Part model, mm, in its own coordinate system. Face numbers are marked on the shaded views. A direction names the side the tool comes from. Round coordinates to 2 decimals unless told otherwise and drop trailing zeros. Write each loop counter-clockwise with the first axis right and the second up, starting at its lowest first coordinate (ties: lowest second). Pieces come first, ordered by that corner, then holes.
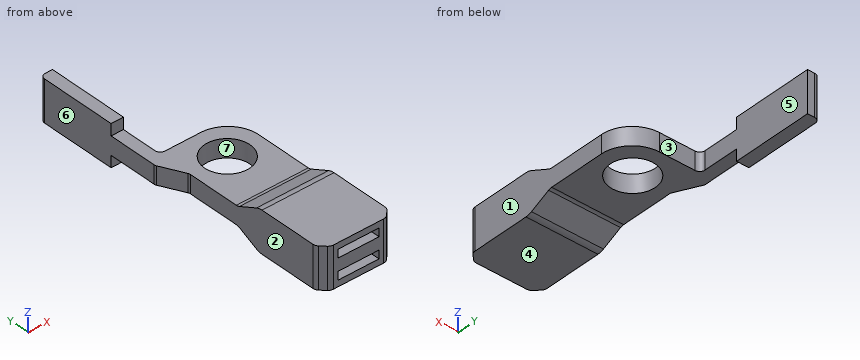
Autodesk Fusion 360 part; units mm, degrees
sketch "Sketch1" plane through (0, 0, 0) normal (0, 0, 1) x (1, 0, 0)
  circle A0 centre (0, 0) radius 11
  line L0 (-17.5, -72.5) -> (17.5, -72.5)
  line L1 (17.5, -72.5) -> (17.5, 17.5)
  line L2 (17.5, 17.5) -> (-17.5, 17.5)
  line L3 (-17.5, 17.5) -> (-17.5, -72.5)
  line L4 (-17.5, 76.6964) -> (-17.5, 51.5115)
  line L5 (-17.5, 51.5115) -> (-17.5, 17.5)
  line L6 (-23.5, 76.6964) -> (-23.5, 13.1317)
  line L7 (-23.5, 13.1317) -> (-17.5, 1.0512)
  line L8 (-17.5, 76.6964) -> (-23.5, 76.6964)
  dimension "d1" = 22
  dimension "d2" = 90
  dimension "d3" = 35
  dimension "d4" = 17.5
  dimension "d10" = 17.5
  dimension "d47" = 6
  dimension "d48" = 6
  dimension "d49" = 6
extrude "Extrude1" add sketch "Sketch1" along normal blind 20
sketch "Sketch4" plane through (-23.5, 0, 0) normal (-1, 0, 0) x (0, -1, 0)
  line L0 (-1.0512, 0) -> (72.5, 0)
  line L1 (72.5, 0) -> (72.5, 20)
  line L2 (72.5, 20) -> (-1.0512, 20)
  line L3 (72.5, 0) -> (72.5, 20)
  line L4 (37.5, 20) -> (25.7892, 14.3853)
  line L5 (25.7892, 14.3853) -> (-37.5, 14.3853)
  line L6 (-37.5, 14.3853) -> (-37.5, 5.6147)
  line L7 (-37.5, 5.6147) -> (25.7892, 5.6147)
  line L8 (25.7892, 5.6147) -> (37.5, 0)
  line L9 (72.5, 0) -> (72.5, 20)
  line L10 (-17.5, 0) -> (72.5, 0)
  line L11 (37.5, 20) -> (72.5, 20)
  line L12 (72.5, 0) -> (37.5, 0)
  line L13 (-37.5, 14.3853) -> (-37.5, 20)
  line L14 (-1.0512, 20) -> (-1.0512, 0)
  line L15 (-37.5, 0) -> (-37.5, 5.6147)
  line L16 (-1.0512, 20) -> (-1.0512, 0)
  line L17 (-76.6964, 0) -> (-13.1317, 0)
  line L18 (-13.1317, 0) -> (-13.1317, 20)
  line L19 (-13.1317, 20) -> (-76.6964, 20)
  line L20 (-76.6964, 20) -> (-76.6964, 0)
  line L21 (-13.1317, 20) -> (-1.0512, 20)
  dimension "d16" = 110
  dimension "d17" = 35
  dimension "d40" = 5.6147
  dimension "d41" = 8.7705
extrude "Extrude2" cut sketch "Sketch4" against normal blind 52 contours L0 L7 L8 L10 L14 L16 | L7 L10 L14 L16 L18 | L7 L10 L15 L17 L18 | L2 L4 L5 L14 L16 | L5 L14 L16 L18 L21 | L5 L13 L18 L19
chamfer "Chamfer1" distance 4 angle 45 2 edges at (-17.5, -72.5, 10) (17.5, -72.5, 10)
sketch "Sketch6" plane through (0, -72.5, 0) normal (0, -1, 0) x (1, 0, 0)
  line L0 (13.5, 0) -> (13.5, 20)
  line L1 (13.5, 20) -> (-13.5, 20)
  line L2 (-13.5, 20) -> (-13.5, 0)
  line L3 (-13.5, 0) -> (13.5, 0)
  line L4 (-10, 17) -> (10, 17)
  line L5 (10, 13) -> (-10, 13)
  line L6 (-10, 13) -> (-10, 17)
  line L7 (10, 3) -> (10, 7)
  line L8 (10, 7) -> (-10, 7)
  line L9 (-10, 7) -> (-10, 3)
  line L10 (-10, 3) -> (10, 3)
  line L11 (10, 17) -> (10, 13)
  dimension "d25" = 20
  dimension "d26" = 4
extrude "Extrude3" cut sketch "Sketch6" against normal blind 30 contours L4 L5 L6 L11 | L7 L8 L9 L10
fillet "Fillet1" radius 4 2 edges at (0, -25.7892, 14.3853) (0, -25.7892, 5.6147)
fillet "Fillet2" radius 7 2 edges at (0, -37.5, 20) (0, -37.5, 0)
fillet "Fillet3" radius 15 1 edges at (17.5, 17.5, 10)
fillet "Fillet4" radius 3 4 edges at (-17.5, -68.5, 10) (-13.5, -72.5, 10) (17.5, -68.5, 10) (13.5, -72.5, 10)
fillet "Fillet6" radius 2.5 3 edges at (-17.5, 1.0512, 10) (-23.5, 13.1317, 10) (-23.5, 76.6964, 10)
fillet "Fillet6" radius 2.5 1 edges at (-17.5, 17.5, 10)
equation "d40 = ( 20 mm - d41 ) / 2"
Q1. Saw through at B-B, the plane z = 10.25. Write the cut outline in (x, y), and give its area (3 significant figures).
Q2. Drop flat-ended pins along their axis: P1, Ø7, axis at x = -8, z = 8.5, coming from the +Y side; P2, Ø3, axis at y = -50, z = 6, coming from the -X side; P3, Ø12.5, axis at x = 6, y = 7, coming from the +Z side. Give the stop position or say it passes through.
Q3. Saw through at C-C, the plane y = -58. Write the cut outline in (x, z), and give its area (3 significant figures).
Q4. Saw through at D-D, the plane y = 8. Write the cut outline in (x, z).
Q5. Wall check: line 1 (Z direction, x = 0.5, y = -44.5); line 2 (X direction, y = 0, z = 10.75); line 3 (Y direction, x = 0, z = 12.5). Give the ranges that are in metal, low to high.
Q6. Two-plate mould, pull along X, no slides. Class the marked faces 4, 5, 6 and 7: released by +X, released by -X, zero draft, split by the parting line, or undercut.
Q7. Tool access for the marked faces 1, 2 and 3: list every direction of +Z, -Z, +X, -X, +Y, -Y with a clear straight run to the whole face (end or side of a thin tool).
Q8. Saw through at A-A, the plane x = 0. Write the cut outline in (y, z), and give its area (3 significant figures).
Computed:
1. outline: (-23.5, 13.72) arc R2.5 ccw to (-23.24, 12.61) - (-17.76, 1.58) arc R2.5 cw to (-17.5, 0.46) - (-17.5, -67.26) arc R3 ccw to (-16.62, -69.38) - (-14.38, -71.62) arc R3 ccw to (-12.26, -72.5) - (12.26, -72.5) arc R3 ccw to (14.38, -71.62) - (16.62, -69.38) arc R3 ccw to (17.5, -67.26) - (17.5, 2.5) arc R15 ccw to (2.5, 17.5) - (-15, 17.5) arc R2.5 cw to (-17.5, 20) - (-17.5, 76.7) - (-21, 76.7) arc R2.5 ccw to (-23.5, 74.2) - close; hole circle Ø22 at (0, 0)
1. area: 3,120 mm2
2. P1: stops at y = 17.5
2. P2: stops at x = -17.5
2. P3: stops at z = 14.39
3. outline: (-17.5, 0) - (17.5, 0) - (17.5, 20) - (-17.5, 20) - close; hole (-10, 3) - (10, 3) - (10, 7) - (-10, 7) - close; hole (-10, 13) - (10, 13) - (10, 17) - (-10, 17) - close
3. area: 540 mm2
4. outline: (-20.95, 5.61) - (-7.55, 5.61) - (-7.55, 14.39) - (-20.95, 14.39) - close; (7.55, 5.61) - (16.46, 5.61) - (16.46, 14.39) - (7.55, 14.39) - close
5. line 1: z = 0 to 3, 7 to 13, 17 to 20
5. line 2: x = -17.5 to -11, 11 to 17.5
5. line 3: y = -72.5 to -11, 11 to 17.5
6. face 4: zero draft
6. face 5: released by +X
6. face 6: released by -X
6. face 7: undercut
7. face 1: +Z, -Z, +X, +Y, -Y
7. face 2: +Z, -Z, -X, -Y
7. face 3: +Z, -Z, +X, +Y
8. outline: (-72.5, 0) - (-39.09, 0) arc R7 ccw to (-36.07, 0.69) - (-26.61, 5.22) arc R4 cw to (-24.88, 5.61) - (-11, 5.61) - (-11, 14.39) - (-24.88, 14.39) arc R4 cw to (-26.61, 14.78) - (-36.07, 19.31) arc R7 ccw to (-39.09, 20) - (-72.5, 20) - (-72.5, 17) - (-42.5, 17) - (-42.5, 13) - (-72.5, 13) - (-72.5, 7) - (-42.5, 7) - (-42.5, 3) - (-72.5, 3) - close; (11, 5.61) - (17.5, 5.61) - (17.5, 14.39) - (11, 14.39) - close
8. area: 815 mm2
